```python
from build123d import *

# Parameters (mm, degrees)
BOSS_EXTRUDE1_DEPTH = 1.3
SKETCH2_W           = 52.88
SKETCH2_H           = 40.08
CUT_EXTRUDE1_DEPTH  = 44.760354203


with BuildPart() as part:
    # Sketch1 → Boss-Extrude1 (new body)
    with BuildSketch(Plane.XY):
        with BuildLine():
            Line((-31.31, 28.35), (31.31, 28.35))
            ThreePointArc((31.31, 28.35), (32.724213562, 27.764213562), (33.31, 26.35))
            Line((33.31, 26.35), (33.31, -21.35))
            ThreePointArc((33.31, -21.35), (31.259747468, -26.299747468), (26.31, -28.35))
            Line((26.31, -28.35), (-31.31, -28.35))
            ThreePointArc((-31.31, -28.35), (-32.724213562, -27.764213562), (-33.31, -26.35))
            Line((-33.31, -26.35), (-33.31, 26.35))
            ThreePointArc((-33.31, 26.35), (-32.724213562, 27.764213562), (-31.31, 28.35))
        make_face()
    extrude(amount=BOSS_EXTRUDE1_DEPTH)

    # Sketch2 → Cut-Extrude1 (cut, through all)
    with BuildSketch(Plane(origin=(0, 0, 0), x_dir=(-1, 0, 0), z_dir=(0, 0, -1))):
        Rectangle(SKETCH2_W, SKETCH2_H)
    extrude(amount=-CUT_EXTRUDE1_DEPTH, mode=Mode.SUBTRACT)


solid = part.part
```
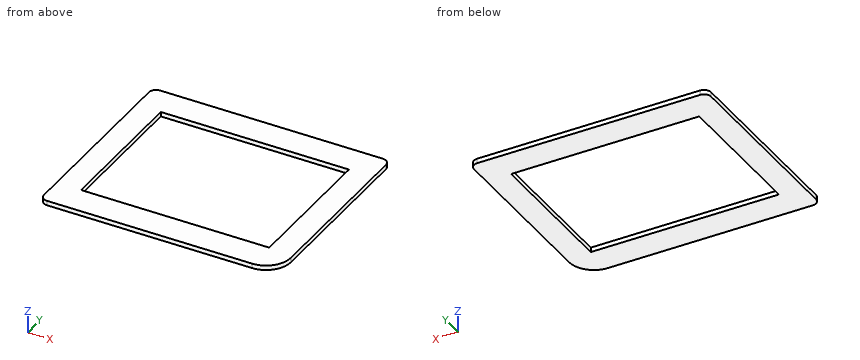
Build history of the part. All positions in model axes, mm. Give positions to 0.01 mm unless a question says otherwise; leave off trailing zeros. Loops run counter-clockwise (first coordinate to the right, second up) from the corner with the lowest first, then second, coordinate; pieces in that order, holes last. Notation, with made-up numbers: (-20, 66.5) -> (-3, 66.5) arc R9 cw to (-3, 73.5) -> close; hole circle Ø4 at (42.25, -27). An arc over 180 degrees is marked (long way). One line per question, with ' | ' between items.
Q1. Cut at C-C, the plane x = -11. Write the cut outline in (y, z), plus the area to 3 significant figures.
Filled sheet:
outline: (-28.35, 0) -> (-20.04, 0) -> (-20.04, 1.3) -> (-28.35, 1.3) -> close; (20.04, 0) -> (28.35, 0) -> (28.35, 1.3) -> (20.04, 1.3) -> close | area: 21.6 mm²
Q2. Drop a flat-ended pin along its axis: pin 1 (8 mm diameter, centred on x = -3, y = 17.5, fed in from +Z). Give the stop position or say it passes through.
Filled sheet:
pin 1: stops at z = 1.3
Q3. Cut at A-A, the plane z = 0.2. Write the cut outline in (x, y).
Filled sheet:
outline: (-33.31, -26.35) arc R2 ccw to (-31.31, -28.35) -> (26.31, -28.35) arc R7 ccw to (33.31, -21.35) -> (33.31, 26.35) arc R2 ccw to (31.31, 28.35) -> (-31.31, 28.35) arc R2 ccw to (-33.31, 26.35) -> close; hole (-26.44, -20.04) -> (26.44, -20.04) -> (26.44, 20.04) -> (-26.44, 20.04) -> close
Q4. Cut at B-B, the plane y = -13.5. Write the cut outline in (x, z).
Filled sheet:
outline: (-33.31, 0) -> (-26.44, 0) -> (-26.44, 1.3) -> (-33.31, 1.3) -> close; (26.44, 0) -> (33.31, 0) -> (33.31, 1.3) -> (26.44, 1.3) -> close
Q5. Drill centre lines: line 1 along X through (y, z) = (-11.5, 0.2); line 2 along Y through (x, z) = (22, 1.25); line 3 along X through (y, z) = (-21.5, 0.7). Where is each one in solid material? Low to high. Write a range as [from, to].
Filled sheet:
line 1: x = [-33.31, -26.44], [26.44, 33.31] | line 2: y = [-28.35, -20.04], [20.04, 28.35] | line 3: x = [-33.31, 33.31]
